Solid Edge part; units mm, degrees
sketch "Sketch1" plane through (0, 0, 0) normal (0, 0, 1) x (1, 0, 0)
  line L0 (4, 0) -> (4, 12)
  line L1 (0, 12) -> (4, 12)
  line L2 (0, 0) -> (0, 12)
  line L3 (0, 0) -> (0, -8)
  line L4 (0, -8) -> (6.5, -8)
  line L5 (6.5, -8) -> (6.5, 0)
  line L6 (6.5, 0) -> (4, 0)
revolve "RevolvedProtrusion1" add sketch "Sketch1" angle 360 about axis through (0, 0, 0) along (0, 1, 0)
sketch "Sketch2" plane through (0, 0, 0) normal (1, 0, 0) x (0, 1, 0)
  line L0 (-8, 3.8415) -> (-4, 3.8415)
  line L1 (-1.7821, 0) -> (-4, 3.8415)
  line L2 (-8, 0) -> (-1.7821, 0)
  line L3 (-8, 0) -> (-8, 3.8415)
revolve "RevolvedCutout1" cut sketch "Sketch2" angle 360 about axis through (0, -4.5, 0) along (0, 1, 0)
sketch "Sketch3" plane through (0, -8, 0) normal (0, -1, 0) x (0, 0, 1)
  circle A0 centre (0, 0) radius 3.8415
  line L0 (-3, -1.7321) -> (0, -3.4641)
  line L1 (0, -3.4641) -> (3, -1.7321)
  line L2 (3, -1.7321) -> (3, 1.7321)
  line L3 (3, 1.7321) -> (0, 3.4641)
  line L4 (0, 3.4641) -> (-3, 1.7321)
  line L5 (-3, 1.7321) -> (-3, -1.7321)
extrude "Protrusion1" add sketch "Sketch3" against normal up to next
sketch "Sketch4" plane through (0, 0, 0) normal (0, 0, 1) x (1, 0, 0)
  line L0 (-3.4641, -8) -> (0, -8)
  line L1 (0, -8) -> (0, -7.0718)
  line L2 (0, -7.0718) -> (-3.4641, -8)
revolve "RevolvedCutout2" cut sketch "Sketch4" angle 360 about axis through (0, -4.5, 0) along (0, 1, 0)
fillet "Round1" radius 0.4 1 edges at (0, 0, -4)
fillet "Round2" radius 0.65 1 edges at (0, -8, -6.5)
chamfer "倒斜角_2" distance 0.5333 angle 45 1 edges at (0, 12, -4)
cosmetic_thread "螺纹_3" thread depth 9.6
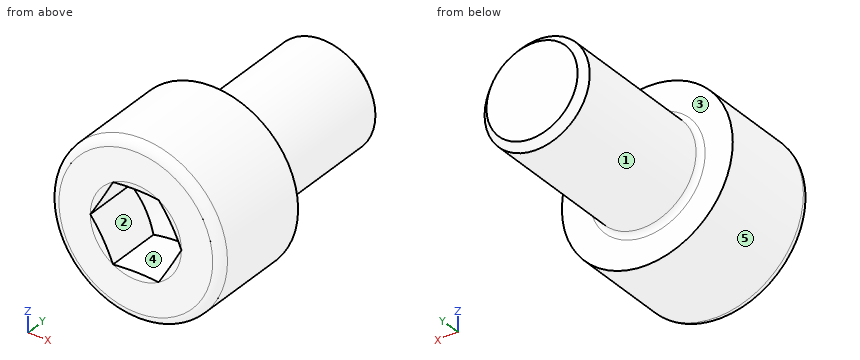
CAD build for the part. Positions are in the model's coordinates, mm. Face numbers are marked on the shaded views. A direction names the side the tool comes from. Coordinates: 2 decimals unless noted, no trailing zeros. Write each loop counter-clockwise with the first axis right and the second up, starting at its lowest first coordinate (ties: lowest second). Pieces come first, ordered by that corner, then holes. Notation, with made-up numbers: (-22, 75) -> (4, 75) arc R30 cw to (4, 97) -> close; hole circle Ø6 at (-24, 13). An arc over 180 degrees is marked (long way). Use CSV: the item, a comma, the result in double quotes. Start each with the question number.
Item 1: Wall check: probe 1 along Y at (x, z) = (-0.75, 4.5); probe 2 along Z at (x, y) = (-3, -7); probe 3 along X at (y, z) = (-4, 5.5). Give the ranges that are in metal, low to high.
Item 2: Drop flat-ended pins along their axis: P1, Ø1.5, axis at x = 2, z = -0.5, coming from the -Y side; P2, Ø2, axis at x = -2.5, z = 4, coming from the +Y side; P3, Ø4, axis at x = 0, z = -0.5, coming from the -Y side; P4, Ø4, axis at x = -0.5, y = -6.5, coming from the +Z side. Give the stop position or say it passes through.
Item 3: Two-plate mould, pull along X, no slides. Class the marked faces 1, 2 and 3: +X half, -X half, draft (parallel to the pull), parting line (faces both ways), or undercut.
Item 4: Tool access for the marked faces 4 and 5: list every direction of +Z, -Z, +X, -X, +Y, -Y with a clear straight run to the whole face (end or side of a thin tool).
Item 5: Band-saw the part on C-C, the plane y = -0.25. Write the cut outline in (x, z).
Item 6: Band-saw the part on A-A, the plane y = -6.5. Write the cut outline in (x, z).
Item 7: Band-saw the part on B-B, the plane y = 8.75. Write the cut outline in (x, z).
Response values:
1,probe 1,"y = -8 to 0"
1,probe 2,"z = -5.77 to -0.8, 0.8 to 5.77"
1,probe 3,"x = -3.46 to 3.46"
2,P1,"stops at y = -3.41"
2,P2,"stops at y = 11.75"
2,P3,"stops at y = -3.23"
2,P4,"stops at z = 6.5"
3,face 1,"parting line"
3,face 2,"undercut"
3,face 3,"draft"
4,face 4,"-Y"
4,face 5,"+Y, -Y"
5,outline,"circle Ø13 at (0, 0)"
6,outline,"circle Ø13 at (0, 0); hole (-3.46, 0) -> (-1.73, -3) -> (1.73, -3) -> (3.46, 0) -> (1.73, 3) -> (-1.73, 3) -> close"
7,outline,"circle Ø8 at (0, 0)"
